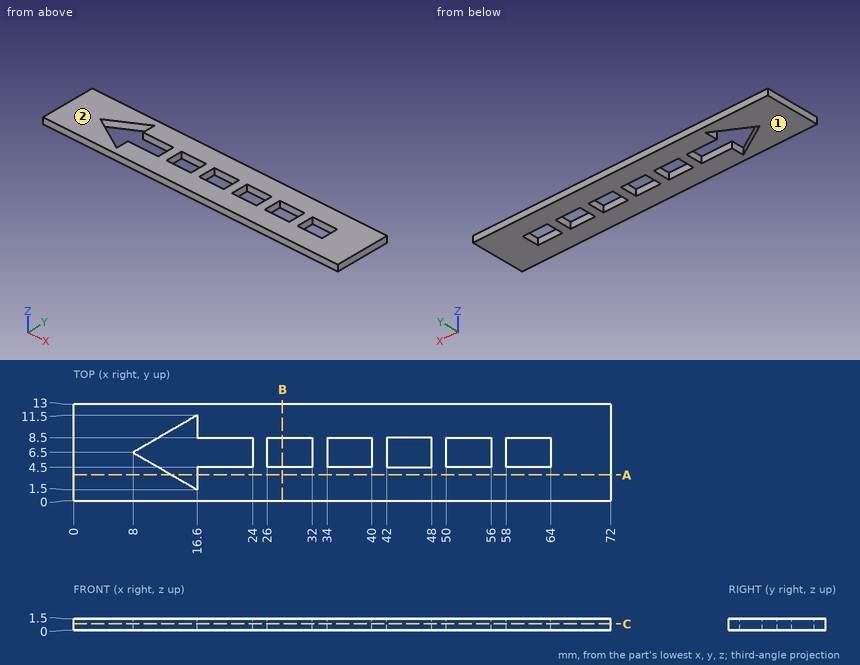
Study the drawing (mm; zero at the part's minimum x, y, z) and answer. Coordinates: 2 decimals unless noted, no trailing zeros. Write each loop counter-clockwise with the first axis right and the second up, starting at its lowest first coordinate (ties: lowest second). Pieces come first, ordered by that corner, then holes. Notation, with made-up numbers: M 30,-36.5 L 81,-36.5 A17 ccw 81,-18.5 Z; hole C -23.5,-21.5 d10. An arc over 180 degrees is marked long. Use a Markdown table: item, result. Add a question column.
1. Section B-B (x = 28) is taken. Give the vertices of the cut face in (y, z).
2. Given P1, Ø6, axis at x = 45, y = 3.5, coming from the -Z side, flat-ended and moving along its own axis, determine where the tip first touches the part or whether it passes through.
3. For a pull along Z with two mould halves and no side action, classify the marked faces 1 and 2 as +Z half, -Z half, draft (parallel to the pull), parting line (faces both ways), or undercut.
4. Section C-C (z = 0.85) is taken. Count the separate pieces of the cut face and the enclosed holes in it, plus the area to 3 significant figures.
5. Section A-A (y = 3.5) is taken. Give the vertices of the cut face in (x, z), plus the area to 3 significant figures.
6. Straight lines are drawn through the part: line 1 along Y through (x, z) = (30, 1.05); line 2 along X through (y, z) = (3.25, 1.3); line 3 along X through (y, z) = (3.5, 0.5). For each, find the intervals that lie inside material, in ascending order. Write a range as [from, to].
Data:
| question | item | result |
|---|---|---|
| 1 | outline | M 0,0 L 4.5,0 L 4.5,1.5 L 0,1.5 Z; M 8.5,0 L 13,0 L 13,1.5 L 8.5,1.5 Z |
| 2 | P1 | stops at z = 0 |
| 3 | face 1 | -Z half |
| 3 | face 2 | +Z half |
| 4 | separate pieces | 1 |
| 4 | enclosed holes | 6 |
| 4 | area | 743 mm2 |
| 5 | outline | M 0,0 L 13.16,0 L 13.16,1.5 L 0,1.5 Z; M 16.6,0 L 72,0 L 72,1.5 L 16.6,1.5 Z |
| 5 | area | 103 mm2 |
| 6 | line 1 | y = [0, 4.5], [8.5, 13] |
| 6 | line 2 | x = [0, 13.59], [16.6, 72] |
| 6 | line 3 | x = [0, 13.16], [16.6, 72] |
